For this review, take the finished solid that the model builds, in its own axes (mm). A direction names the side the tool comes from. Round coordinates to 2 decimals unless told otherwise and drop trailing zeros. Order: outer loops, then holes, each group sorted by start corner. A loop starts at its lowest first (then second) coordinate and runs counter-clockwise, first axis right, second up. Notation, with made-up numbers: M 84.25,74.25 L 108.25,74.25 A28 cw 108.25,113.25 Z; hole C -30.75,35 d8. An arc over 180 degrees is marked long. Put each result on its own line as item: value.
from build123d import *

# Parameters (mm, degrees)
SKETCH1_W           = 14.732
SKETCH1_H           = 9.144
SKETCH1_W_2         = 1.778
SKETCH1_H_2         = 5.08
BOSS_EXTRUDE1_DEPTH = 2.032
SKETCH2_W           = 3.048
SKETCH2_H           = 9.144
BOSS_EXTRUDE2_DEPTH = 1.016
SKETCH3_R           = 1.016
CUT_EXTRUDE1_DEPTH  = 10.144


with BuildPart() as part:
    # Sketch1 → Boss-Extrude1 (new body)
    with BuildSketch(Plane(origin=(0, 0, 0), x_dir=(1, 0, 0), z_dir=(0, 1, 0))):
        Rectangle(SKETCH1_W, SKETCH1_H)
        with Locations((4.445, 0)):
            Rectangle(SKETCH1_W_2, SKETCH1_H_2, mode=Mode.SUBTRACT)
    extrude(amount=BOSS_EXTRUDE1_DEPTH)

    # Sketch2 → Boss-Extrude2 (add)
    with BuildSketch(Plane(origin=(0, 2.032, 0), x_dir=(1, 0, 0), z_dir=(0, 1, 0))):
        with Locations((-5.842, 0)):
            Rectangle(SKETCH2_W, SKETCH2_H)
    extrude(amount=BOSS_EXTRUDE2_DEPTH)

    # Sketch3 → Cut-Extrude1 (cut, through all)
    with BuildSketch(Plane.XY.offset(4.572)):
        with Locations((-5.842, 2.286)):
            Circle(SKETCH3_R)
    extrude(amount=-CUT_EXTRUDE1_DEPTH, mode=Mode.SUBTRACT)


solid = part.part
(1) Add section B-B on z = 0. Give the boundary of the cut face in (x, y), then the cut area to 3 significant figures.
A:
outline: M -7.37,0 L 3.56,0 L 3.56,2.03 L -4.32,2.03 L -4.32,3.05 L -5.17,3.05 A1.02 cw long -6.51,3.05 L -7.37,3.05 Z; M 5.33,0 L 7.37,0 L 7.37,2.03 L 5.33,2.03 Z
area: 26.4 mm2
(2) Add section D-D on y = 0.55. Give the boundary of the cut face in (x, z).
A:
outline: M -7.37,-4.57 L 7.37,-4.57 L 7.37,4.57 L -7.37,4.57 Z; hole M 3.56,-2.54 L 5.33,-2.54 L 5.33,2.54 L 3.56,2.54 Z
(3) Draft analysis for pull direction Z (two halves, no side actions). For faces 1 (the face through (3.556, 1, 0)), 2 (the face through (0, 0, 0)), 3 (the face through (0, 1, 4.572)), state which applies: released by +Z, released by -Z, zero draft, split by the parting line, or undercut.
A:
face 1: undercut
face 2: zero draft
face 3: released by +Z
(4) Insertion check: pin 1 Ø0.8 at (y, z) = (2.5, 1) entering from +X; pin 2 Ø1.6 at (x, y) = (-5.842, 2.286) entering from +Z. Each pin has a flat end and moves straight along its axis. Give the tip position at first contact, or say it passes through.
A:
pin 1: stops at x = -4.32
pin 2: passes through
(5) For faces 4 (the face through (-7.366, 2, 0)), 5 (the face through (5.334, 1, 0)), 6 (the face through (-4.318, 2.5, 0.1)), list the 3-axis set-ups (+Z, -Z, +X, -X, +Y, -Y) from which the entire face can be reached by the end or side of a thin tool; tool diameter is ignored.
A:
face 4: +Z, -Z, -X, +Y, -Y
face 5: +Y, -Y
face 6: +Z, -Z, +X, +Y
(6) To check wall thickness, follow L1, parallel to X at y = 0.2, z = 0.5; L2, parallel to Z at x = 4.5, y = 0.9; L3, parallel to X at y = 2.3, z = -0.5. State the ranges of each line that lie inside material, in increasing order.
A:
L1: x = -7.37 to 3.56, 5.33 to 7.37
L2: z = -4.57 to -2.54, 2.54 to 4.57
L3: x = -7.37 to -6.86, -4.83 to -4.32
(7) Add section A-A on y = 1.85. Give the boundary of the cut face in (x, z), then the cut area to 3 significant figures.
A:
outline: M -7.37,-4.57 L -6.76,-4.57 L -6.76,4.57 L -7.37,4.57 Z; M -4.92,-4.57 L 7.37,-4.57 L 7.37,4.57 L -4.92,4.57 Z; hole M 3.56,-2.54 L 5.33,-2.54 L 5.33,2.54 L 3.56,2.54 Z
area: 109 mm2
(8) Add section C-C on z = -3. Give the boundary of the cut face in (x, y).
A:
outline: M -7.37,0 L 7.37,0 L 7.37,2.03 L -4.32,2.03 L -4.32,3.05 L -5.17,3.05 A1.02 cw long -6.51,3.05 L -7.37,3.05 Z
